Geometry check sheet. Reference: drawing and pictorial views, mm from the part's lowest x, y, z. A direction names the side the tool comes from. Round coordinates to 2 decimals unless told otherwise and drop trailing zeros. Order: outer loops, then holes, each group sorted by start corner. A loop starts at its lowest first (then second) coordinate and runs counter-clockwise, first axis right, second up.
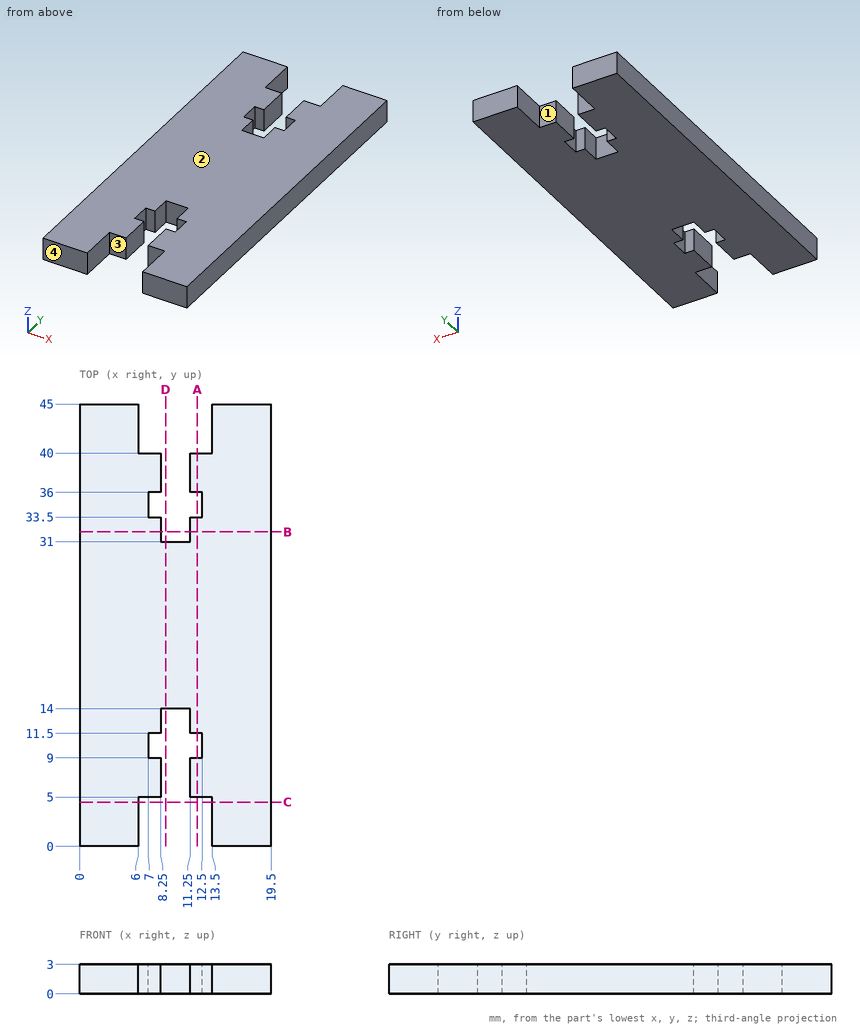
1) Sectioned sample at C-C on y = 4.5. Record the cut outline in (x, z).
2) Scan lines: probe 1 along X at (y, z) = (38, 0.9); probe 2 along Y at (x, z) = (6.75, 0.9); probe 3 along Y at (x, z) = (10.5, 2.8). Record each from-to range of solid material in increasing order.
3) Sectioned sample at D-D on x = 8.75. Record the cut outline in (y, z).
4) Tool access check on the marked faces 1 and 2. Record the directions out of +Z, -Z, +X, -X, +Y, -Y that give a thin tool (end or side, any length) a straight path to the whole face; none if there is none.
5) Sectioned sample at A-A on x = 12. Record the cut outline in (y, z).
6) Sectioned sample at B-B on y = 32. Record the cut outline in (x, z), then the cut area to 3 significant figures.
7) Go/stop test with flat-tipped pins: pin 1 Ø1 at (x, z) = (11.5, 1) entering from -Y; pin 2 Ø1.4 at (x, z) = (11.5, 1) entering from +Y; pin 3 Ø1.5 at (x, z) = (9.5, 1) entering from +Y. Record where each tip stops, or that it passes through.
8) Draft check along X on the marked faces 3 and 4. Enter one of: released by +X, released by -X, zero draft, split by the parting line, or undercut.
Returned:
1. outline: (0, 0) - (6, 0) - (6, 3) - (0, 3) - close; (13.5, 0) - (19.5, 0) - (19.5, 3) - (13.5, 3) - close
2. probe 1: x = 0 to 8.25, 11.25 to 19.5
2. probe 2: y = 5 to 40
2. probe 3: y = 14 to 31
3. outline: (14, 0) - (31, 0) - (31, 3) - (14, 3) - close
4. face 1: +Z, -Z, +Y
4. face 2: +Z, +X, -X, +Y, -Y
5. outline: (5, 0) - (9, 0) - (9, 3) - (5, 3) - close; (11.5, 0) - (33.5, 0) - (33.5, 3) - (11.5, 3) - close; (36, 0) - (40, 0) - (40, 3) - (36, 3) - close
6. outline: (0, 0) - (8.25, 0) - (8.25, 3) - (0, 3) - close; (11.25, 0) - (19.5, 0) - (19.5, 3) - (11.25, 3) - close
6. area: 49.5 mm2
7. pin 1: stops at y = 5
7. pin 2: stops at y = 40
7. pin 3: stops at y = 31
8. face 3: undercut
8. face 4: zero draft
